Can you work these out from the model? Positions are in its coordinate system, mm. Coordinates: 2 decimals unless noted, no trailing zeros. Loops run counter-clockwise (first coordinate to the right, second up) from the corner with the lowest first, then second, coordinate; pieces in that order, holes last.
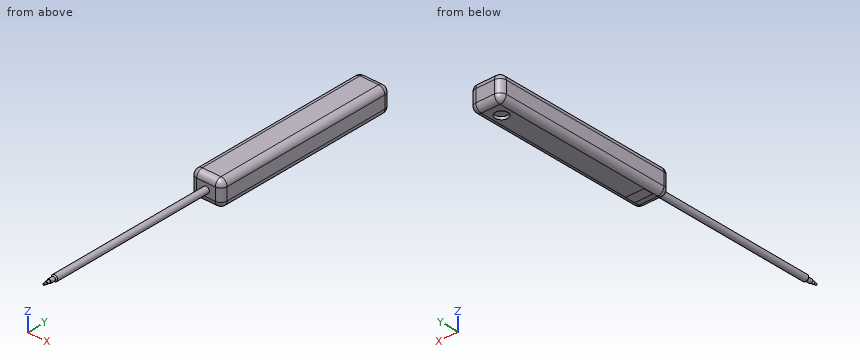
```python
from build123d import *

# Parameters (mm, degrees)
F0_W         = 25.4
F0_H         = 20.32
F1_DEPTH     = 127
F2_R         = 5.08
F3_R         = 5.08
F4_R         = 5.08
F5_DEPTH     = 25.4
F6_R         = 2.54
F7_DEPTH     = 139.192
F8_R         = 5.08
F9_R         = 1.6125595219
F10_DEPTH    = 2.54
F11_R        = 1.0795
F12_DEPTH    = 2.54
F13_R        = 0.680816043
F14_DEPTH    = 2.286
F15_S5_R     = 1.6125595219
F15_T6_DEPTH = 5
F16_R        = 5.1312830473
F17_DEPTH    = 2.286
F18_W        = 15.1486136019
F18_H        = 8.2696229219
F19_DEPTH    = 0.00254


# Not quite as in the source:
# - a fillet or chamfer that OpenCascade refuses, or shapes differently, is made with other operations: its cross-section is extruded or revolved along the edge and cut away or added


with BuildPart() as f1:
    # F0 (on Front) → F1 (new body)
    with BuildSketch(Plane.XZ):
        with Locations((-0.1826275468, -0.0669072086)):
            Rectangle(F0_W, F0_H)
    extrude(amount=F1_DEPTH)

    # F2
    f2_edges = [f1.edges().sort_by_distance(p)[0] for p in [
        (12.517372, -63.5, 10.093093),
        (12.517372, -63.5, -10.226907),
    ]]
    fillet(f2_edges, radius=F2_R)

    # F3
    f3_edges = [f1.edges().sort_by_distance(p)[0] for p in [
        (-12.882628, -63.5, -10.226907),
    ]]
    fillet(f3_edges, radius=F3_R)

    # F4
    f4_edges = [f1.edges().sort_by_distance(p)[0] for p in [
        (-12.882628, -63.5, 10.093093),
        (-12.882628, 0, 2.473093),
    ]]
    fillet(f4_edges, radius=F4_R)

    # F5 (add): a face of the model
    f5_faces = [f1.faces().sort_by_distance(p)[0] for p in [
        (-0.1826275468, -127, -0.0669072086),
    ]]
    extrude(f5_faces, amount=F5_DEPTH)

    # F6 (on face) → F7 (join)
    with BuildSketch(Plane.XZ.offset(152.4)):
        Circle(F6_R)
    extrude(amount=F7_DEPTH)

    # F8
    f8_edges = [f1.edges().sort_by_distance(p)[0] for p in [
        (-0.182628, -152.4, 10.093093),
        (-0.182628, -152.4, -10.226907),
        (12.517372, -152.4, -0.066907),
        (-12.882628, -152.4, -0.066907),
    ]]
    fillet(f8_edges, radius=F8_R)

    # F9 (on face) → F10 (join)
    with BuildSketch(Plane.XZ.offset(291.592)):
        Circle(F9_R)
    extrude(amount=F10_DEPTH)

    # F11 (on face) → F12 (join)
    with BuildSketch(Plane.XZ.offset(294.132)):
        Circle(F11_R)
    extrude(amount=F12_DEPTH)

    # F13 (on face) → F14 (join)
    with BuildSketch(Plane.XZ.offset(296.672)):
        Circle(F13_R)
    extrude(amount=F14_DEPTH)

    # F15: chamfer of 2.286 on 1 edges, made by hand


with BuildPart() as f15_tool2:
    # F15_s3 → F15_t4 (revolve)
    with BuildSketch(Plane.XY):
        Polygon((2.54, -289.306), (0.254, -291.592), (2.54, -291.592), align=None)
    revolve(axis=Axis((0, -291.592, 0), (0, -1, 0)))

    # F15_s5 → F15_t6 (cut, symmetric)
    with BuildSketch(Plane.XZ.offset(290.4)):
        Circle(F15_S5_R)
    extrude(amount=F15_T6_DEPTH, both=True, mode=Mode.SUBTRACT)


with BuildPart() as f1_1:
    add(f1.part)

    # F15_t1: cut F15_tool2
    add(f15_tool2.part, mode=Mode.SUBTRACT)

    # F16 (on face) → F17 (cut)
    with BuildSketch(Plane(origin=(0, 0, -10.2269072086), x_dir=(1, 0, 0), z_dir=(0, 0, -1))):
        with Locations((0, 15.0263812393)):
            Circle(F16_R)
    extrude(amount=-F17_DEPTH, mode=Mode.SUBTRACT)

    # F18 (on face) → F19 (join)
    with BuildSketch(Plane(origin=(0, 0, -10.2269072086), x_dir=(1, 0, 0), z_dir=(0, 0, -1))):
        with Locations((0.0473735854, 139.4127830863)):
            Rectangle(F18_W, F18_H)
    extrude(amount=F19_DEPTH)


solid = f1_1.part
```
(1) If I drill on probe 1 along Z at (x, y) = (7.75, -23.5); probe 2 along Y at (x, z) = (1.25, -5.25); probe 3 along Y at (x, z) = (0, -9.25), over which ranges is the centre line in solid material (lowest first)?
Check values:
probe 1: z = -10.22 to 10.08
probe 2: y = -152.4 to 0
probe 3: y = -150.32 to -20.16, -9.9 to -2.08
(2) I want a section at B-B on y = -184. Write out the boundary of the cut face in (x, z).
Check values:
outline: circle Ø5.08 at (0, 0)
(3) I'm going to push flat-ended pins straight in: pin 1 (7.5 mm diameter, centred on x = 0, y = -68, fed in from -Z); pin 2 (5 mm diameter, centred on x = 0, y = -14, fed in from -Z); pin 3 (2 mm diameter, centred on y = -218, z = -3, fed in from -X). Where does each tip first touch, or does it pass through?
Check values:
pin 1: stops at z = -10.23
pin 2: stops at z = -7.94
pin 3: stops at x = -1.57
(4) I want a section at A-A on y = -27.5. Write out the boundary of the cut face in (x, z).
Check values:
outline: (-12.88, -5.15) arc R5.08 ccw to (-7.8, -10.23) - (7.44, -10.23) arc R5.08 ccw to (12.52, -5.15) - (12.52, 5.01) arc R5.08 ccw to (7.44, 10.09) - (-7.8, 10.09) arc R5.08 ccw to (-12.88, 5.01) - close
